Autodesk Inventor part; units mm, degrees
ref_plane "YZ Plane" through (0, 0, 0) normal (1, 0, 0) x (0, 1, 0)
ref_plane "XZ Plane" through (0, 0, 0) normal (0, 1, 0) x (-1, 0, 0)
ref_plane "XY Plane" through (0, 0, 0) normal (0, 0, 1) x (1, 0, 0)
sketch "Sketch1" plane through (0, 0, 0) normal (0, 1, 0) x (-1, 0, 0)
  line L0 (0, 0) -> (51.38, 0)
  line L1 (51.38, 0) -> (51.38, -40)
  line L2 (51.38, -40) -> (0, -40)
  line L3 (0, -40) -> (0, 0)
  dimension "d0" = 51.38
  dimension "d1" = 40
extrude "Extrusion1" add sketch "Sketch1" along normal blind 65
sketch "Sketch2" plane through (-51.38, 0, 0) normal (0, 0, 1) x (1, 0, 0)
  line L0 (51.38, 0) -> (0, 0)
  line L1 (0, 0) -> (-20, 0)
  line L2 (-20, 0) -> (-20, 3)
  line L3 (-20, 3) -> (0, 3)
  line L4 (0, 3) -> (0, 0)
  line L5 (51.38, 65) -> (0, 65)
  line L6 (0, 65) -> (-20, 65)
  line L7 (-20, 65) -> (-20, 62)
  line L8 (-20, 62) -> (0, 62)
  line L9 (0, 62) -> (0, 65)
  dimension "d4" = 20
  dimension "d5" = 3
  dimension "d6" = 20
  dimension "d7" = 3
extrude "Extrusion2" add sketch "Sketch2" against normal blind 40
properties part number "motor_support"
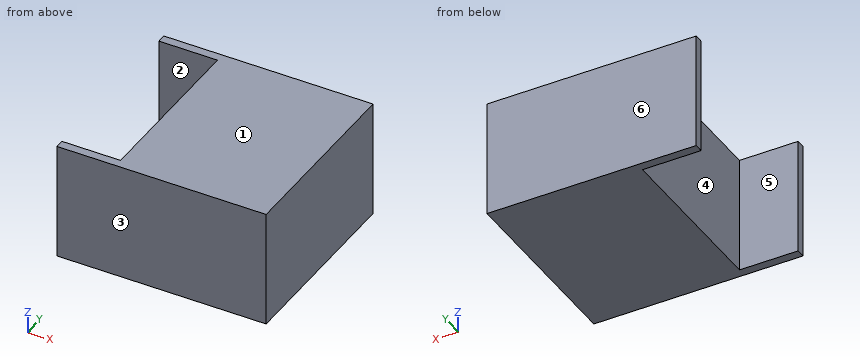
Verification items for the finished model (mm, model axes). Face numbers are marked on the shaded views. A direction names the side the tool comes from. Give positions to 0.01 mm unless a question says otherwise; leave off trailing zeros. Loops run counter-clockwise (first coordinate to the right, second up) from the corner with the lowest first, then second, coordinate; pieces in that order, holes last. Notation, with made-up numbers: (-11, 55) - (15, 55) arc R20 ccw to (15, 80) - close; hole circle Ø3 at (71, 8). An arc over 180 degrees is marked (long way). Write each question's results on one line, items separated by ' | '.
1) Depth check by flat-ended pin: P1, Ø5, axis at x = -48.5, z = -17, coming from the -Y side. Enter the tip coordinate at first touch or a pass-through.
Solution:
P1: y = 0
2) Sectioned sample at A-A on x = -60.5. Record the boundary of the cut face in (y, z), plus the area to 3 significant figures.
Solution:
outline: (0, -40) - (3, -40) - (3, 0) - (0, 0) - close; (62, -40) - (65, -40) - (65, 0) - (62, 0) - close | area: 240 mm2
3) Sectioned sample at B-B on z = -28. Record the boundary of the cut face in (x, y).
Solution:
outline: (-71.38, 0) - (0, 0) - (0, 65) - (-71.38, 65) - (-71.38, 62) - (-51.38, 62) - (-51.38, 3) - (-71.38, 3) - close
4) Tool access check on the marked faces 5 and 6. Record the directions out of +Z, -Z, +X, -X, +Y, -Y that give a thin tool (end or side, any length) a straight path to the whole face; none if there is none.
Solution:
face 5: +Z, -Z, -X | face 6: +Z, -Z, +X, -X, +Y
5) Mould release check, pull along Y, two halves, no side actions. Record for the marked faces 1, 2, 3 and 4: pulls with the +Y half, pulls with the -Y half, needs draft (parallel to the pull), parting line crosses it, or undercut.
Solution:
face 1: needs draft | face 2: undercut | face 3: pulls with the -Y half | face 4: undercut
6) Material ranges on L1, parallel to Y at x = -66, z = -26.5; L2, parallel to X at y = 16, z = -27, recorded low to high. Write a range as from..to.
Solution:
L1: 0..3, 62..65 | L2: -51.38..0
7) Sectioned sample at C-C on y = 54.5. Record the boundary of the cut face in (x, z).
Solution:
outline: (-51.38, -40) - (0, -40) - (0, 0) - (-51.38, 0) - close
